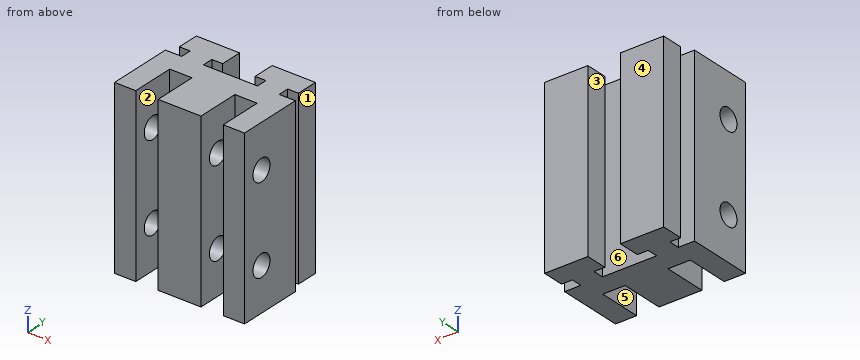
```python
from build123d import *

# Parameters (mm, degrees)
SKETCH2_W             = 9.9
SKETCH2_H             = 40
BOSS_EXTRUDE1_DEPTH   = 10
SKETCH2_W_2           = 4.9
BOSS_EXTRUDE1_2_DEPTH = 10
BOSS_EXTRUDE1_3_DEPTH = 10
SKETCH3_R             = 2.5
CUT_EXTRUDE1_DEPTH    = 30
SKETCH4_W             = 30
SKETCH4_H             = 40
BOSS_EXTRUDE2_DEPTH   = 5
BOSS_EXTRUDE3_DEPTH   = 40


with BuildPart() as part:
    # Sketch2 → Boss-Extrude1 (new body)
    with BuildSketch(Plane(origin=(0, 0, 0), x_dir=(1, 0, 0), z_dir=(0, 1, 0))):
        Rectangle(SKETCH2_W, SKETCH2_H)
    extrude(amount=BOSS_EXTRUDE1_DEPTH)


with BuildPart() as body_2:
    # Sketch2 → Boss-Extrude1 2 (new body)
    with BuildSketch(Plane(origin=(0, 0, 0), x_dir=(1, 0, 0), z_dir=(0, 1, 0))):
        with Locations((-12.55, 0)):
            Rectangle(SKETCH2_W_2, SKETCH2_H)
    extrude(amount=BOSS_EXTRUDE1_2_DEPTH)


with BuildPart() as body_3:
    # Sketch2 → Boss-Extrude1 3 (new body)
    with BuildSketch(Plane(origin=(0, 0, 0), x_dir=(1, 0, 0), z_dir=(0, 1, 0))):
        with Locations((12.55, 0)):
            Rectangle(SKETCH2_W_2, SKETCH2_H)
    extrude(amount=BOSS_EXTRUDE1_3_DEPTH)


with BuildPart() as cut_extrude1_tool:
    # Sketch3 → Cut-Extrude1 (new body)
    with BuildSketch(Plane.ZY.offset(15)):
        with Locations((-10, 5)):
            Circle(SKETCH3_R)
        with Locations((10, 5)):
            Circle(SKETCH3_R)
    extrude(amount=-CUT_EXTRUDE1_DEPTH)


with BuildPart() as part_1:
    add(part.part)

    # Cut-Extrude1: cut by cut_extrude1_tool
    add(cut_extrude1_tool.part, mode=Mode.SUBTRACT)



with BuildPart() as body_2_1:
    add(body_2.part)

    # Cut-Extrude1: cut by cut_extrude1_tool
    add(cut_extrude1_tool.part, mode=Mode.SUBTRACT)


with BuildPart() as body_3_1:
    add(body_3.part)

    # Cut-Extrude1: cut by cut_extrude1_tool
    add(cut_extrude1_tool.part, mode=Mode.SUBTRACT)


with BuildPart() as part_2:
    add(part_1.part)

    add(body_2_1.part)  # Boss-Extrude2 merges body 2

    add(body_3_1.part)  # Boss-Extrude2 merges body 3
    # Sketch4 → Boss-Extrude2 (add)
    with BuildSketch(Plane(origin=(0, 10, 0), x_dir=(1, 0, 0), z_dir=(0, 1, 0))):
        Rectangle(SKETCH4_W, SKETCH4_H)
    extrude(amount=BOSS_EXTRUDE2_DEPTH)

    # Sketch5 → Boss-Extrude3 (add)
    with BuildSketch(Plane.XY.offset(20)):
        Polygon((-11.25, 15), (-11.25, 17.5), (-13.75, 17.5), (-13.75, 22.5), (-3.75, 22.5), (-3.75, 17.5), (-6.25, 17.5), (-6.25, 15), align=None)
    boss_extrude3 = extrude(amount=-BOSS_EXTRUDE3_DEPTH)

    # Mirror1: Boss-Extrude3 across Right Plane
    add(boss_extrude3.mirror(Plane(origin=(0, 0, 0), x_dir=(0, 0, -1), z_dir=(1, 0, 0))))


solid = part_2.part
```
The model under review builds one solid part; all positions refer to its coordinate system, in mm. Face numbers are marked on the shaded views. A direction names the side the tool comes from. Round coordinates to 2 decimals unless told otherwise and drop trailing zeros. Write each loop counter-clockwise with the first axis right and the second up, starting at its lowest first coordinate (ties: lowest second). Pieces come first, ordered by that corner, then holes. Notation, with made-up numbers: M 80,39 L 98,39 A21 ccw 98,63 Z; hole C 21,81 d3. An arc over 180 degrees is marked long. Use CSV: the item, a comma, the result in double quotes. Start each with the question number.
(1) We need section A-A, the plane z = 3.5. State the section outline as (x, y) points.
(2) Clearance check with flat-ended pins moving along their axes: P1, Ø5, axis at x = 10, y = 4.5, coming from the -Z side; P2, Ø4, axis at y = 5, z = 10, coming from the -X side; P3, Ø0.8, axis at x = -5.5, z = -6, coming from the -Y side; P4, Ø3, axis at y = 17, z = -8, coming from the -X side. State where each tip first meets the part, or that it passes through.
(3) We need section D-D, the plane z = -10. State how many separate pieces and enclosed holes the cut face has, then the cut area to 4 significant figures.
(4) The part is to be moulded in two halves that separate along Y. For the marked faces 4, 5 and 6, say which applies: +Y half, -Y half, draft (parallel to the pull), parting line (faces both ways), or undercut.
(5) For line 1 along X through (y, z) = (5.75, 17.5); line 2 along Y through (x, z) = (-12.5, 10), list the stretches that pass through material, from the lowest coordinate up.
(6) We need section C-C, the plane y = 20.25. State the section outline as (x, z) points, then the cut area to 3 significant figures.
(7) We need section B-B, the plane x = -5.75. State the section outline as (y, z) points, then the cut area to 3 significant figures.
(8) Tool access review of the marked faces 1, 2 and 3: name each direction out of +Z, -Z, +X, -X, +Y, -Y from which nothing blocks a thin tool from reaching the whole face with its end or side.
Findings:
1,outline,"M -15,0 L -10.1,0 L -10.1,10 L -4.95,10 L -4.95,0 L 4.95,0 L 4.95,10 L 10.1,10 L 10.1,0 L 15,0 L 15,15 L 11.25,15 L 11.25,17.5 L 13.75,17.5 L 13.75,22.5 L 3.75,22.5 L 3.75,17.5 L 6.25,17.5 L 6.25,15 L -6.25,15 L -6.25,17.5 L -3.75,17.5 L -3.75,22.5 L -13.75,22.5 L -13.75,17.5 L -11.25,17.5 L -11.25,15 L -15,15 Z"
2,P1,"z = -20"
2,P2,"through"
2,P3,"y = 10"
2,P4,"x = -13.75"
3,separate pieces,"4"
3,enclosed holes,"0"
3,area,"373.5 mm^2"
4,face 4,"+Y half"
4,face 5,"draft"
4,face 6,"undercut"
5,line 1,"-15 to -10.1, -4.95 to 4.95, 10.1 to 15"
5,line 2,"0 to 2.5, 7.5 to 15, 17.5 to 22.5"
6,outline,"M -13.75,-20 L -3.75,-20 L -3.75,20 L -13.75,20 Z; M 3.75,-20 L 13.75,-20 L 13.75,20 L 3.75,20 Z"
6,area,"800 mm^2"
7,outline,"M 10,-20 L 15,-20 L 15,20 L 10,20 Z; M 17.5,-20 L 22.5,-20 L 22.5,20 L 17.5,20 Z"
7,area,"400 mm^2"
8,face 1,"+Z, -Z, +X, +Y"
8,face 2,"+Z, -Z, -Y"
8,face 3,"+Z, -Z, +Y"
